from build123d import *

# Parameters (mm, degrees)
ESQUISSE1_R        = 1.65
BOSS_EXTRU_1_DEPTH = 1.4


with BuildPart() as part:
    # Esquisse1 → Boss.-Extru.1 (new, symmetric)
    with BuildSketch(Plane.XY):
        with BuildLine():
            Line((0, -5), (40, -5))
            Line((40, -5), (40, 5))
            Line((40, 5), (0, 5))
            ThreePointArc((0, 5), (-5, 0), (0, -5))
        make_face()
        Circle(ESQUISSE1_R, mode=Mode.SUBTRACT)
    extrude(amount=BOSS_EXTRU_1_DEPTH, both=True)


solid = part.part
Can you work these out from the model? Positions are in its coordinate system, mm. Round coordinates to 2 decimals unless told otherwise and drop trailing zeros. Loops run counter-clockwise (first coordinate to the right, second up) from the corner with the lowest first, then second, coordinate; pieces in that order, holes last. Notation, with made-up numbers: (30, 61.5) - (38, 61.5) arc R28 cw to (38, 99.5) - close; hole circle Ø6 at (-22.5, 85.25). An arc over 180 degrees is marked (long way). Write item = value, one per line. Start each with the question number.
(1) If we section it at C-C (z = -0.2): Please give me the cut outline in (x, y).
(2) If we mould it in two halves opening along Y, with no side actions, what happens to faces 1 (the face through (-5, 0, 0)), 2 (the face through (17, 0, 1.4)), 3 (the face through (-1.216, 1.115, -0.02))? For each: released by +Y, released by -Y, zero draft, split by the parting line, or undercut.
(3) If I drill on probe 1 along Y at (x, z) = (0, -0.8); probe 2 along X at (y, z) = (-0.5, 0.3); probe 3 along X at (y, z) = (-1.5, 1.3), over which ranges is the centre line in solid material (lowest first)? Write a range as [from, to].
(4) If we section it at B-B (x = -1): Please give me the cut outline in (y, z).
(5) If we section it at D-D (y = 4.25): Please give me the cut outline in (x, z).
(6) If we section it at A-A (y = 0): Please give me the cut outline in (x, z), and give its area (3 significant figures).
Ans:
q1.outline = (0, -5) - (40, -5) - (40, 5) - (0, 5) arc R5 ccw to start; hole circle Ø3.3 at (0, 0)
q2.face_1 = split by the parting line
q2.face_2 = zero draft
q2.face_3 = undercut
q3.probe_1 = [-5, -1.65], [1.65, 5]
q3.probe_2 = [-4.97, -1.57], [1.57, 40]
q3.probe_3 = [-4.77, -0.69], [0.69, 40]
q4.outline = (-4.9, -1.4) - (-1.31, -1.4) - (-1.31, 1.4) - (-4.9, 1.4) - close; (1.31, -1.4) - (4.9, -1.4) - (4.9, 1.4) - (1.31, 1.4) - close
q5.outline = (-2.63, -1.4) - (40, -1.4) - (40, 1.4) - (-2.63, 1.4) - close
q6.outline = (-5, -1.4) - (-1.65, -1.4) - (-1.65, 1.4) - (-5, 1.4) - close; (1.65, -1.4) - (40, -1.4) - (40, 1.4) - (1.65, 1.4) - close
q6.area = 117 mm²
